The listing builds one solid part. Answer for the finished solid, in the listing's coordinates (mm). Coordinates: 2 decimals unless noted, no trailing zeros. Order: outer loops, then holes, each group sorted by start corner. A loop starts at its lowest first (then second) coordinate and runs counter-clockwise, first axis right, second up. Notation, with made-up numbers: (4.25, 74.25) -> (49.25, 74.25) arc R22 ccw to (49.25, 109.25) -> close; hole circle Ø8 at (81.5, -16). An arc over 180 degrees is marked (long way). Answer in a Markdown table with one row per item. Add a question column.
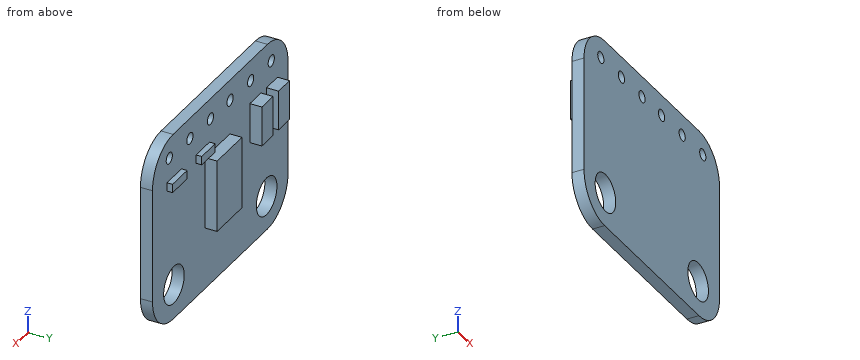
```python
from build123d import *

# Parameters (mm, degrees)
BOSS_EXTRUDE1_DEPTH = 0.8128
SKETCH2_R           = 0.381
SKETCH2_R_2         = 1.27
CUT_EXTRUDE1_DEPTH  = 0.8128
SKETCH4_W           = 3.069128824
SKETCH4_H           = 4.866519185
SKETCH4_W_2         = 1.37347754
SKETCH4_H_2         = 2.696085542
SKETCH4_W_3         = 1.356521027
SKETCH4_H_3         = 2.679129029
BOSS_EXTRUDE2_DEPTH = 0.8128
SKETCH4_3_W         = 1.661738258
SKETCH4_3_H         = 0.576521436
SKETCH4_3_W_2       = 1.797390361
BOSS_EXTRUDE3_DEPTH = 0.381


with BuildPart() as part:
    # Sketch1 → Boss-Extrude1 (new body)
    with BuildSketch(Plane(origin=(0, 0, 0), x_dir=(1, 0, 0), z_dir=(0, 1, 0))):
        with BuildLine():
            Line((5.8166, 6.3881), (-5.8166, 6.3881))
            ThreePointArc((-5.8166, 6.3881), (-7.612651224, 5.644151224), (-8.3566, 3.8481))
            Line((-8.3566, 3.8481), (-8.3566, -3.8481))
            ThreePointArc((-8.3566, -3.8481), (-7.612651224, -5.644151224), (-5.8166, -6.3881))
            Line((-5.8166, -6.3881), (5.8166, -6.3881))
            ThreePointArc((5.8166, -6.3881), (7.612651224, -5.644151224), (8.3566, -3.8481))
            Line((8.3566, -3.8481), (8.3566, 3.8481))
            ThreePointArc((8.3566, 3.8481), (7.612651224, 5.644151224), (5.8166, 6.3881))
        make_face()
    extrude(amount=BOSS_EXTRUDE1_DEPTH)

    # Sketch2 → Cut-Extrude1 (cut)
    with BuildSketch(Plane(origin=(0, 0.8128, 0), x_dir=(1, 0, 0), z_dir=(0, 1, 0))):
        with Locations(Location((-1.2065, -4.993693032, 0), (0, 0, 270))):
            Circle(SKETCH2_R)
        with Locations(Location((-5.715, 4.061084825, 0), (0, 0, 270))):
            Circle(SKETCH2_R_2)
        with Locations(Location((-3.7465, -4.993693032, 0), (0, 0, 270))):
            Circle(SKETCH2_R)
        with Locations(Location((-6.2865, -4.993693032, 0), (0, 0, 270))):
            Circle(SKETCH2_R)
        with Locations(Location((6.2865, -4.993693032, 0), (0, 0, 90))):
            Circle(SKETCH2_R)
        with Locations(Location((3.7465, -4.993693032, 0), (0, 0, 90))):
            Circle(SKETCH2_R)
        with Locations(Location((5.715, 4.061084825, 0), (0, 0, 90))):
            Circle(SKETCH2_R_2)
        with Locations(Location((1.2065, -4.993693032, 0), (0, 0, 90))):
            Circle(SKETCH2_R)
    extrude(amount=-CUT_EXTRUDE1_DEPTH, mode=Mode.SUBTRACT)

    # Sketch4 → Boss-Extrude2 (add)
    with BuildSketch(Plane(origin=(0, 0.8128, 0), x_dir=(1, 0, 0), z_dir=(0, 1, 0))):
        with Locations((0.347608513, -0.237391179)):
            Rectangle(SKETCH4_W, SKETCH4_H)
        with Locations((-4.332389031, -2.102607592)):
            Rectangle(SKETCH4_W_2, SKETCH4_H_2)
        with Locations((-6.375648829, -2.111085849)):
            Rectangle(SKETCH4_W_3, SKETCH4_H_3)
    extrude(amount=BOSS_EXTRUDE2_DEPTH)

    # Sketch4<3> → Boss-Extrude3 (add)
    with BuildSketch(Plane(origin=(0, 0.8128, 0), x_dir=(1, 0, 0), z_dir=(0, 1, 0))):
        with Locations((2.153477131, -3.162389645)):
            Rectangle(SKETCH4_3_W, SKETCH4_3_H)
        with Locations((5.680431802, -3.162389645)):
            Rectangle(SKETCH4_3_W_2, SKETCH4_3_H)
    extrude(amount=BOSS_EXTRUDE3_DEPTH)


solid = part.part
```
Q1. A cutting plane is placed at D-D (z = 5). Determine the outline of the cut face in (x, y), then the cut area to 3 significant figures.
Q2. Given pin 1 (0.7 mm diameter, centred on x = -6.5, y = 1, fed in from -Z); pin 2 (0.9 mm diameter, centred on x = 1, y = 1.5, fed in from -Z); pin 3 (0.7 mm diameter, centred on x = -4.5, y = 1.5, fed in from -Z), each flat-ended and moving along its own axis, determine where each tip first touches the part or whether it passes through.
Q3. A cutting plane is placed at B-B (z = 1.75). Determine the outline of the cut face in (x, y), then the cut area to 3 significant figures.
Q4. A cutting plane is placed at C-C (y = 0.5). State how many separate pieces and enclosed holes the cut face has, then the cut area to 3 significant figures.
Q5. Straight lines are drawn through the part: line 1 (Z direction, x = 6.5, y = 0.2); line 2 (Y direction, x = -3.75, z = -2.5); line 3 (X direction, y = 0.85, z = 2.75). For each, find the intervals that lie inside material, in ascending order.
Q6. A cutting plane is placed at A-A (z = -4.25). Determine the outline of the cut face in (x, y).
Returned:
| question | item | result |
|---|---|---|
| 1 | outline | (-8.08, 0) -> (-6.67, 0) -> (-6.67, 0.81) -> (-8.08, 0.81) -> close; (-5.91, 0) -> (-4.13, 0) -> (-4.13, 0.81) -> (-5.91, 0.81) -> close; (-3.37, 0) -> (-1.59, 0) -> (-1.59, 0.81) -> (-3.37, 0.81) -> close; (-0.83, 0) -> (0.83, 0) -> (0.83, 0.81) -> (-0.83, 0.81) -> close; (1.59, 0) -> (3.37, 0) -> (3.37, 0.81) -> (1.59, 0.81) -> close; (4.13, 0) -> (5.91, 0) -> (5.91, 0.81) -> (4.13, 0.81) -> close; (6.67, 0) -> (8.08, 0) -> (8.08, 0.81) -> (6.67, 0.81) -> close |
| 1 | area | 9.42 mm² |
| 2 | pin 1 | stops at z = -6.36 |
| 2 | pin 2 | stops at z = -2.2 |
| 2 | pin 3 | stops at z = 0.75 |
| 3 | outline | (-8.36, 0) -> (8.36, 0) -> (8.36, 0.81) -> (1.88, 0.81) -> (1.88, 1.63) -> (-1.19, 1.63) -> (-1.19, 0.81) -> (-3.65, 0.81) -> (-3.65, 1.63) -> (-5.02, 1.63) -> (-5.02, 0.81) -> (-5.7, 0.81) -> (-5.7, 1.63) -> (-7.05, 1.63) -> (-7.05, 0.81) -> (-8.36, 0.81) -> close |
| 3 | area | 18.3 mm² |
| 4 | separate pieces | 1 |
| 4 | enclosed holes | 8 |
| 4 | area | 195 mm² |
| 5 | line 1 | z = -6.29 to -5.06, -3.06 to 4.68, 5.31 to 6.29 |
| 5 | line 2 | y = 0 to 0.81 |
| 5 | line 3 | x = -7.05 to -5.7, -5.02 to -3.65 |
| 6 | outline | (-8.32, 0) -> (-6.97, 0) -> (-6.97, 0.81) -> (-8.32, 0.81) -> close; (-4.46, 0) -> (4.46, 0) -> (4.46, 0.81) -> (-4.46, 0.81) -> close; (6.97, 0) -> (8.32, 0) -> (8.32, 0.81) -> (6.97, 0.81) -> close |
